from build123d import *

# Parameters (mm, degrees)
SKETCH_1_R          = 15.5
EXTRUDE_1_DEPTH     = 3
SKETCH_2_R          = 14.5
EXTRUDE_2_DEPTH     = 1
SKETCH_3_R          = 12.3
EXTRUDE_3_DEPTH     = 12.5
SKETCH_4_W          = 15
SKETCH_4_H          = 6.5
CUT_EXTRUDE_1_DEPTH = 10
EXTRUDE_START       = 5
EXTRUDE_4_DEPTH     = 5
SKETCH_6_W          = 15
SKETCH_6_H          = 7
EXTRUDE_5_DEPTH     = 10


with BuildPart() as part:
    # ｽｹｯﾁ1 → ﾎﾞｽ - 押し出し1 (new body)
    with BuildSketch(Plane.XY):
        Circle(SKETCH_1_R)
    extrude(amount=EXTRUDE_1_DEPTH)

    # ｽｹｯﾁ2 → ﾎﾞｽ - 押し出し2 (add)
    with BuildSketch(Plane.XY.offset(3)):
        Circle(SKETCH_2_R)
    extrude(amount=EXTRUDE_2_DEPTH)

    # ｽｹｯﾁ3 → ﾎﾞｽ - 押し出し3 (add)
    with BuildSketch(Plane.XY.offset(4)):
        Circle(SKETCH_3_R)
    extrude(amount=EXTRUDE_3_DEPTH)

    # ｽｹｯﾁ4 → ｶｯﾄ - 押し出し1 (cut)
    with BuildSketch(Plane.XY.offset(16.5)):
        Rectangle(SKETCH_4_W, SKETCH_4_H)
    extrude(amount=-CUT_EXTRUDE_1_DEPTH, mode=Mode.SUBTRACT)

    # ｽｹｯﾁ5 → ﾎﾞｽ - 押し出し4 (add)
    with BuildSketch(Plane(origin=(0, 0, 0), x_dir=(-1, 0, 0), z_dir=(0, 0, -1)).offset(EXTRUDE_START)):
        with BuildLine():
            Line((-12.158947323, -7.9), (12.158947323, -7.9))
            ThreePointArc((12.158947323, -7.9), (14.5, 0), (12.158947323, 7.9))
            Line((12.158947323, 7.9), (-12.158947323, 7.9))
            ThreePointArc((-12.158947323, 7.9), (-14.5, 0), (-12.158947323, -7.9))
        make_face()
    extrude(amount=-EXTRUDE_4_DEPTH)

    # ｽｹｯﾁ6 → ﾎﾞｽ - 押し出し5 (add)
    with BuildSketch(Plane(origin=(0, 0, -5), x_dir=(-1, 0, 0), z_dir=(0, 0, -1))):
        Rectangle(SKETCH_6_W, SKETCH_6_H)
    extrude(amount=EXTRUDE_5_DEPTH)


solid = part.part
Work out the finished part from the listing and answer in its coordinate system (mm). A direction names the side the tool comes from. Round coordinates to 2 decimals unless told otherwise and drop trailing zeros. Write each loop counter-clockwise with the first axis right and the second up, starting at its lowest first coordinate (ties: lowest second). Pieces come first, ordered by that corner, then holes. Notation, with made-up numbers: (41.5, -16) -> (56.5, -16) arc R28 cw to (56.5, 21) -> close; hole circle Ø9 at (79, 8). An arc over 180 degrees is marked (long way). Write each question's results on one line, items separated by ' | '.
Item 1: The mould has two halves that part along X. Classify faces 4 (the face through (0, 0, -15)), 5 (the face through (7.5, 0, 12)), 6 (the face through (14.5, 0.1, -2.5)): +X half, -X half, draft (parallel to the pull), parting line (faces both ways), or undercut.
Result set:
face 4: draft | face 5: undercut | face 6: +X half
Item 2: A cutting plane is placed at B-B, the plane y = 0. Determine the outline of the cut face in (x, z), plus the area to 4 significant figures.
Result set:
outline: (-15.5, 0) -> (-14.5, 0) -> (-14.5, -5) -> (-7.5, -5) -> (-7.5, -15) -> (7.5, -15) -> (7.5, -5) -> (14.5, -5) -> (14.5, 0) -> (15.5, 0) -> (15.5, 3) -> (14.5, 3) -> (14.5, 4) -> (12.3, 4) -> (12.3, 16.5) -> (7.5, 16.5) -> (7.5, 6.5) -> (-7.5, 6.5) -> (-7.5, 16.5) -> (-12.3, 16.5) -> (-12.3, 4) -> (-14.5, 4) -> (-14.5, 3) -> (-15.5, 3) -> close | area: 574.5 mm^2
Item 3: A cutting plane is placed at A-A, the plane z = 14. Determine the outline of the cut face in (x, y), plus the area to 3 significant figures.
Result set:
outline: circle Ø24.6 at (0, 0); hole (-7.5, -3.25) -> (7.5, -3.25) -> (7.5, 3.25) -> (-7.5, 3.25) -> close | area: 378 mm^2
Item 4: Which of the six approach directions +Z, -Z, +X, -X, +Y, -Y give full straight-line access (tool end or side, diameter ignored) to faces 1 (the face through (0, 3.5, -10)), 2 (the face through (0, -7.9, -3)), 3 (the face through (6.691, -12.864, 3.493))?
Result set:
face 1: -Z, +X, -X, +Y | face 2: -Z, +X, -X, -Y | face 3: +Z
Item 5: Find the intervals of material crossed by line 1 along Z through (x, y) = (-12.5, -5); line 2 along Y through (x, z) = (-4.5, 7.5); line 3 along Z through (x, y) = (1, 8.5), in increasing order. Write a range as [from, to].
Result set:
line 1: [-5, 4] | line 2: [-11.45, -3.25], [3.25, 11.45] | line 3: [0, 16.5]
Item 6: Flat-ended cylindrical pins translate along their axes: P1, Ø2, axis at y = -7, z = 6.5, coming from the -X side; P2, Ø7.5, axis at y = 0.5, z = -10, coming from the -X side; P3, Ø7, axis at y = 1.5, z = 13, coming from the +X side. Find the tip coordinate at first contact, or state that the pin passes through.
Result set:
P1: x = -10.74 | P2: x = -7.5 | P3: x = 12.3
Item 7: A cutting plane is placed at D-D, the plane z = 5. Determine the outline of the cut face in (x, y).
Result set:
outline: circle Ø24.6 at (0, 0)
Item 8: A cutting plane is placed at C-C, the plane x = 0. Determine the outline of the cut face in (y, z), plus the area to 4 significant figures.
Result set:
outline: (-15.5, 0) -> (-7.9, 0) -> (-7.9, -5) -> (-3.5, -5) -> (-3.5, -15) -> (3.5, -15) -> (3.5, -5) -> (7.9, -5) -> (7.9, 0) -> (15.5, 0) -> (15.5, 3) -> (14.5, 3) -> (14.5, 4) -> (12.3, 4) -> (12.3, 16.5) -> (3.25, 16.5) -> (3.25, 6.5) -> (-3.25, 6.5) -> (-3.25, 16.5) -> (-12.3, 16.5) -> (-12.3, 4) -> (-14.5, 4) -> (-14.5, 3) -> (-15.5, 3) -> close | area: 513.5 mm^2
